Can you work these out from the model? Positions are in its coordinate system, mm. A direction names the side the tool comes from. Give positions to 0.01 mm unless a question says otherwise; leave off trailing zeros. Order: outer loops, then holes, each group sorted by start corner. A loop starts at its lowest first (then second) coordinate and runs counter-clockwise, first axis right, second up. Notation, with made-up numbers: (-23.5, -25.5) - (-7.5, -25.5) arc R28 cw to (-7.5, 3.5) - close; hole circle Ø4 at (-40, 35). An arc over 180 degrees is marked (long way). Return JSON: item names as keys, results as strings.
Autodesk Inventor part; units mm, degrees
ref_plane "YZ Plane" through (0, 0, 0) normal (1, 0, 0) x (0, 1, 0)
ref_plane "XZ Plane" through (0, 0, 0) normal (0, 1, 0) x (-1, 0, 0)
ref_plane "XY Plane" through (0, 0, 0) normal (0, 0, 1) x (1, 0, 0)
sketch "Sketch1" plane through (0, 0, 0) normal (0, 1, 0) x (-1, 0, 0)
  line L0 (50, -50) -> (-50, -50)
  line L1 (-50, -50) -> (-50, 50)
  line L2 (-50, 50) -> (50, 50)
  line L3 (50, 50) -> (50, -50)
  point P0 (0, 0)
  point P1 (-50, 0)
  point P2 (0, -50)
  dimension "d0" = 100
  dimension "d1" = 100
extrude "Extrusion1" add sketch "Sketch1" along normal blind 18
sketch "Sketch2" plane through (0, 18, 0) normal (0, 1, 0) x (1, 0, 0)
  line L0 (-50, 50) -> (-32, 50) construction
  line L1 (50, 50) -> (-50, 50) construction
  line L2 (50, 50) -> (-50, 50) construction
  line L3 (-50, 50) -> (-50, -50) construction
  line L4 (-50, -50) -> (50, -50) construction
  line L5 (50, -50) -> (50, 50) construction
  line L6 (50, -50) -> (50, -32) construction
  line L7 (-32, 50) -> (50, -32)
  line L8 (50, -32) -> (50, 50)
  line L9 (50, 50) -> (-32, 50)
  point P0 (0, 0)
  point P1 (-41, 50)
  point P2 (0, 50)
  point P3 (-50, 0)
  point P4 (0, -50)
  point P5 (50, -41)
  point P6 (50, 0)
  dimension "d4" = 18
  dimension "d5" = 18
extrude "Extrusion2" cut sketch "Sketch2" against normal blind 18
sketch "Sketch3" plane through (0, 18, 0) normal (0, 1, 0) x (1, 0, 0)
  line L0 (-50, 0) -> (-32, 0)
  line L1 (-32, 0) -> (-32, -50)
  line L2 (-32, -50) -> (-50, -50)
  line L3 (-50, -50) -> (-50, 0)
  line L4 (50, -32) -> (-32, 50)
  line L5 (-32, 50) -> (-50, 50)
  line L6 (-50, 50) -> (-50, -50)
  line L7 (-50, -50) -> (50, -50)
  line L8 (50, -50) -> (50, -32)
  line L9 (-50, 50) -> (-50, -50)
  line L10 (-50, -32) -> (0, -32)
  line L11 (0, -32) -> (0, -50)
  line L12 (0, -50) -> (-50, -50)
  line L13 (-50, -50) -> (-50, -32)
  line L14 (-50, -50) -> (50, -50)
  point P0 (0, 0)
  point P1 (-41, -50)
  point P2 (-50, -25)
  point P3 (-50, 0)
  point P4 (-41, 0)
  point P5 (-50, 0)
  point P6 (-25, -50)
  point P7 (0, -50)
  point P8 (-50, -41)
  point P9 (0, -41)
  point P10 (0, -50)
  dimension "d8" = 18
  dimension "d9" = 18
extrude "Extrusion3" cut sketch "Sketch3" against normal blind 18 contours L0 L1 L10 L3 | L10 L1 L2 L3 | L10 L11 L7 L1
sketch "Sketch4" plane through (0, 18, 0) normal (0, 1, 0) x (1, 0, 0)
  line L0 (0, -32) -> (0, -50)
  line L1 (0, -50) -> (50, -50)
  line L2 (50, -50) -> (50, -32)
  line L3 (50, -32) -> (-32, 50)
  line L4 (-32, 50) -> (-50, 50)
  line L5 (-50, 50) -> (-50, 0)
  line L6 (-50, 0) -> (-32, 0)
  line L7 (-32, 0) -> (-32, -32)
  line L8 (-32, -32) -> (0, -32)
  point P0 (0, 0)
  point P1 (-32, -3.175)
  point P2 (-3.175, -32)
  point P3 (-16, -32)
  dimension "d12" = 3.175
  dimension "d13" = 3.175
hole "Hole1" at (-32, 18, 3.175) at (-3.175, 18, 32) direction (0, -1, 0) diameter 6.35 end through all
sketch "Sketch5" plane through (0, 18, 0) normal (0, 1, 0) x (1, 0, 0)
  arc A0 (-32, -6.35) -> (-32, 0) centre (-32, -3.175) ccw
  line L0 (-32, -6.35) -> (-32, -32)
  line L1 (-32, -32) -> (-6.35, -32)
  arc A1 (0, -32) -> (-6.35, -32) centre (-3.175, -32) ccw
  line L2 (0, -32) -> (0, -50)
  line L3 (0, -50) -> (50, -50)
  line L4 (50, -50) -> (50, -32)
  line L5 (50, -32) -> (-32, 50)
  line L6 (-32, 50) -> (-50, 50)
  line L7 (-50, 50) -> (-50, 0)
  line L8 (-50, 0) -> (-32, 0)
  point P0 (0, 0)
  point P1 (-41, 25)
  point P2 (25, -41)
  point P3 (-50, 25)
  point P4 (-41, 50)
  point P5 (0, -41)
  point P6 (25, -50)
hole "Hole2" at (-41, 18, -25) at (25, 18, 41) direction (0, -1, 0) diameter 6.35 end through all
equation "\"d0\" = legBaseWidth"
equation "\"d1\" = legBaseWidth"
equation "\"d2\" = plyThickness"
equation "\"d4\" = plyThickness"
equation "\"d5\" = d4"
equation "\"d6\" = plyThickness"
equation "\"d8\" = plyThickness"
equation "\"d9\" = d8"
equation "\"d10\" = plyThickness"
equation "\"d14\" = millDiameter"
equation "\"d21\" = millDiameter"
equation "\"plyThickness\" = 18"
equation "\"legHeight\" = 702"
equation "\"legBaseWidth\" = 100"
equation "\"millDiameter\" = 6.35"
equation "\"legTopTabHeight\" = 18"
equation "\"legTopSlotDepth\" = 49"
properties part number "foot"
1. Thinking about a two-plate mould opening in X: for faces 3 (the face through (8, 9, -10)), 4 (the face through (-41, 9, 0)), 5 (the face through (-28.826, 8.874, 3.105)), 6 (the face through (26.22, 8.87, 43.93)), which applies, +X half, -X half, draft (parallel to the pull), parting line (faces both ways), or undercut?
Checks:
{"face 3": "+X half", "face 4": "draft", "face 5": "-X half", "face 6": "undercut"}
2. On a 3-axis mill with a long thin cutter (end or side, diameter ignored), from which of +Z, -Z, +X, -X, +Y, -Y can I reach the whole of each face in a straight line? I mean faces 1 (the face through (-19, 9, 32)), 2 (the face through (-3.245, 8.874, 28.826)). Say none if no direction works.
Checks:
{"face 1": "+Z, -X, +Y, -Y", "face 2": "+Z, +Y, -Y"}
3. Suppose I cut it at B-B (x = -41). List the corners of the cut face in (y, z) for me (3 decimals), plus the area to 3 significant figures.
Checks:
{"outline": "(0, -50) - (18, -50) - (18, -28.175) - (0, -28.175) - close; (0, -21.825) - (18, -21.825) - (18, 0) - (0, 0) - close", "area": "786 mm^2"}
4. Suppose I cut it at C-C (y = 5.5). List the corners of the cut face in (x, z) for me (3 decimals).
Checks:
{"outline": "(-50, -50) - (-32, -50) - (50, 32) - (50, 50) - (0, 50) - (0, 32) arc R3.175 cw to (-6.35, 32) - (-32, 32) - (-32, 6.35) arc R3.175 cw to (-32, 0) - (-50, 0) - close; hole circle Ø6.35 at (-41, -25); hole circle Ø6.35 at (25, 41)"}
5. For pin 1 Ø10 at (y, z) = (3.5, -5.5) entering from +X; pin 2 Ø1 at (y, z) = (15, -33.5) entering from +X; pin 3 Ø9 at (x, y) = (-43.5, 5.5) entering from +Z, each with a flat end and sliding along its axis, tell me the tip position at first contact or that it passes through.
Checks:
{"pin 1": "x = 17.5", "pin 2": "x = -15", "pin 3": "z = 0"}
6. If I drill on L1, parallel to X at y = 14.75, z = 41 (3 decimals); L2, parallel to X at y = 4.75, z = 34; L3, parallel to Z at x = -37, y = 14, over which ranges is the centre line in solid material (lowest first)? Write a range as [from, to].
Checks:
{"L1": "[0, 21.825], [28.175, 50]", "L2": "[0, 50]", "L3": "[-50, 0]"}
7. Suppose I cut it at D-D (x = 35.5). List the corners of the cut face in (y, z) for me.
Checks:
{"outline": "(0, 17.5) - (18, 17.5) - (18, 50) - (0, 50) - close"}
8. Suppose I cut it at A-A (z = 41). List the corners of the cut face in (x, y) for me (3 decimals), plus the area to 3 significant figures.
Checks:
{"outline": "(0, 0) - (21.825, 0) - (21.825, 18) - (0, 18) - close; (28.175, 0) - (50, 0) - (50, 18) - (28.175, 18) - close", "area": "786 mm^2"}
